Input: part model. Units: mm. Frame: model coordinates. A direction names the side the tool comes from. Give positions to 0.01 mm unless a question says otherwise; leave off trailing zeros. Loops run counter-clockwise (first coordinate to the right, second up) from the corner with the lowest first, then second, coordinate; pieces in that order, holes last. Notation, with made-up numbers: (23, 24.25) -> (32, 24.25) arc R27 cw to (32, 44.25) -> close; hole circle Ø4 at (29.25, 4.5). An arc over 180 degrees is marked (long way). Answer as a JSON object with one key per item and string values.
```python
from build123d import *

# Parameters (mm, degrees)
EXTRUDE1_DEPTH     = 53
HOLE1_D            = 9
HOLE1_DEPTH        = 53
SKETCH5_R          = 4
CUT_EXTRUDE1_DEPTH = 4
SKETCH6_R          = 5.5
CUT_EXTRUDE2_DEPTH = 3
SKETCH7_R          = 2
CUT_EXTRUDE3_DEPTH = 33
CUT_EXTRUDE4_DEPTH = 5


with BuildPart() as part:
    # Sketch1 → Extrude1 (new body)
    with BuildSketch(Plane(origin=(0, 0, 0), x_dir=(1, 0, 0), z_dir=(0, 1, 0))):
        with BuildLine():
            Line((-37.947331922, 31), (37.947331922, 31))
            ThreePointArc((37.947331922, 31), (49, 0), (37.947331922, -31))
            Line((37.947331922, -31), (-37.947331922, -31))
            ThreePointArc((-37.947331922, -31), (-49, 0), (-37.947331922, 31))
        make_face()
    extrude(amount=EXTRUDE1_DEPTH)

    # Sketch2 → Revolve1 (revolve)
    with BuildSketch(Plane.XY, mode=Mode.PRIVATE) as revolve1_sk:
        Polygon((0, 89), (-6.75, 89), (-6.75, 75), (-18, 75), (-18, 74), (-30.95, 74), (-30.95, 53), (0, 53), align=None)
    revolve(revolve1_sk.sketch.rotate(Axis((0, 0, 0), (0, 1, 0)), 270), axis=Axis((0, 0, 0), (0, 1, 0)))  # turned: the seam where the file's is

    # Hole1
    with Locations(Plane(origin=(0, 53, 0), x_dir=(-1, 0, 0), z_dir=(0, 1, 0))):
        with Locations((40, 0), (-40, 0)):
            Hole(HOLE1_D / 2, depth=HOLE1_DEPTH)

    # Sketch5 → Cut-Extrude1 (cut)
    with BuildSketch(Plane.XZ):
        with Locations(Location((0, 0, 0), (0, 0, 270))):  # turned: the seam where the file's is
            Circle(SKETCH5_R)
    extrude(amount=-CUT_EXTRUDE1_DEPTH, mode=Mode.SUBTRACT)

    # Sketch6 → Cut-Extrude2 (cut)
    with BuildSketch(Plane.XZ):
        with Locations(Location((31, -13, 0), (0, 0, 270))):  # turned: the seam where the file's is
            Circle(SKETCH6_R)
    extrude(amount=-CUT_EXTRUDE2_DEPTH, mode=Mode.SUBTRACT)

    # Sketch7 → Cut-Extrude3 (cut)
    with BuildSketch(Plane.XZ.offset(-3)):
        with Locations(Location((31, -13, 0), (0, 0, 270))):  # turned: the seam where the file's is
            Circle(SKETCH7_R)
    extrude(amount=-CUT_EXTRUDE3_DEPTH, mode=Mode.SUBTRACT)

    # Sketch8 → Cut-Revolve1 (revolve, cut)
    with BuildSketch(Plane(origin=(0, 0, 0), x_dir=(0.920504853, 0, -0.390731128), z_dir=(0.390731128, 0, 0.920504853)), mode=Mode.PRIVATE) as cut_revolve1_sk:
        Polygon((49, 28), (47, 28), (47, 33.4215), (45.517364509, 34.2775), (32, 34.2775), (32, 40), (49, 40), align=None)
    revolve(cut_revolve1_sk.sketch.rotate(Axis((47.484793311, 40, -20.156098913), (-0.920504853, 0, 0.390731128)), 270), axis=Axis((47.484793311, 40, -20.156098913), (-0.920504853, 0, 0.390731128)), mode=Mode.SUBTRACT)  # turned: the seam where the file's is

    # Sketch9 → Revolve2 (revolve)
    with BuildSketch(Plane(origin=(0, 0, 0), x_dir=(0.920504853, 0, -0.390731128), z_dir=(0.390731128, 0, 0.920504853)), mode=Mode.PRIVATE) as revolve2_sk:
        Polygon((47, 31), (47, 34.2775), (38, 34.2775), (37, 35.2775), (37, 40), (52, 40), (52, 31), align=None)
    revolve(revolve2_sk.sketch.rotate(Axis((53.930450878, 40, -22.892118224), (-0.920504853, 0, 0.390731128)), 270), axis=Axis((53.930450878, 40, -22.892118224), (-0.920504853, 0, 0.390731128)))  # turned: the seam where the file's is

    # Sketch10 → Cut-Extrude4 (cut)
    with BuildSketch(Plane(origin=(47.86625238, 0, -20.318018681), x_dir=(-0.390731128, 0, -0.920504853), z_dir=(0.920504853, 0, -0.390731128))):
        Polygon((4.041451884, 40), (2.020725942, 43.5), (-2.020725942, 43.5), (-4.041451884, 40), (-2.020725942, 36.5), (2.020725942, 36.5), align=None)
    extrude(amount=-CUT_EXTRUDE4_DEPTH, mode=Mode.SUBTRACT)


solid = part.part
```
Q1. Section C-C, the plane x = -40. Return the cut outline in (y, z), then the cut area to 3 significant figures.
Evaluation:
{"outline": "(0, -28.3) -> (53, -28.3) -> (53, -4.5) -> (0, -4.5) -> close; (0, 4.5) -> (53, 4.5) -> (53, 28.3) -> (0, 28.3) -> close", "area": "2,520 mm2"}
Q2. Pin query (flat end, axial travel): pin 1 (10 mm diameter, centred on x = 31, z = -13, fed in from +Y); pin 2 (5.5 mm diameter, centred on x = 32, z = -12.5, fed in from -Y); pin 3 (5.5 mm diameter, centred on x = -40, z = 0, fed in from +Y); pin 4 (4.5 mm diameter, centred on x = 31, z = -13, fed in from +Y). Return the tip coordinate at first contact, or that it passes through.
Evaluation:
{"pin 1": "stops at y = 74", "pin 2": "stops at y = 3", "pin 3": "passes through", "pin 4": "stops at y = 53"}
Q3. Access query for faces 4 (the flat face through (44.407, 41.726, -22.158)), 5 (the flat face through (28.6, 3, -12.9)), 6 (the flat face through (43.286, 40.049, -18.312)), 7 (the cylindrical face through (6.59, 81.9, 1.46)), 8 (the cylindrical face through (-35.708, 26.129, 1.352)). Directions: +Z, -Z, +X, -X, +Y, -Y. A direction counts if a zero-diameter tool reaches every point of the face in a straight line with its end or side. Return the directions, or none.
Evaluation:
{"face 4": "+X", "face 5": "-Y", "face 6": "none", "face 7": "+Y", "face 8": "+Y, -Y"}
Q4. Section D-D, the plane z = 21. Return the cut outline in (x, y), then the cut area to 3 significant figures.
Evaluation:
{"outline": "(-44.27, 0) -> (44.27, 0) -> (44.27, 53) -> (22.74, 53) -> (22.74, 74) -> (-22.74, 74) -> (-22.74, 53) -> (-44.27, 53) -> close", "area": "5,650 mm2"}
Q5. Section B-B, the plane x = 0. Return the cut outline in (y, z).
Evaluation:
{"outline": "(0, -31) -> (53, -31) -> (53, -30.95) -> (74, -30.95) -> (74, -18) -> (75, -18) -> (75, -6.75) -> (89, -6.75) -> (89, 6.75) -> (75, 6.75) -> (75, 18) -> (74, 18) -> (74, 30.95) -> (53, 30.95) -> (53, 31) -> (0, 31) -> (0, 4) -> (4, 4) -> (4, -4) -> (0, -4) -> close"}
Q6. Section A-A, the plane z = 0. Return the cut outline in (x, y).
Evaluation:
{"outline": "(-49, 0) -> (-44.5, 0) -> (-44.5, 53) -> (-49, 53) -> close; (-35.5, 0) -> (-4, 0) -> (-4, 4) -> (4, 4) -> (4, 0) -> (35.5, 0) -> (35.5, 53) -> (30.95, 53) -> (30.95, 74) -> (18, 74) -> (18, 75) -> (6.75, 75) -> (6.75, 89) -> (-6.75, 89) -> (-6.75, 75) -> (-18, 75) -> (-18, 74) -> (-30.95, 74) -> (-30.95, 53) -> (-35.5, 53) -> close; (44.5, 0) -> (49, 0) -> (49, 53) -> (44.5, 53) -> close"}
Q7. Ray query, line 1 along X through (y, z) = (32, -0.5); line 2 along Z through (x, y) = (31, 28); line 3 along Y through (x, z) = (-32, -2.5). Return the intervals inside material, ascending.
Evaluation:
{"line 1": "x = -49 to -44.47, -35.53 to 35.53, 44.47 to 49", "line 2": "z = -31 to -15, -11 to 31", "line 3": "y = 0 to 53"}
Q8. Draft query along Y for faces 1 (the flat face through (0, 89, 0)), 2 (the cylindrical face through (45.991, 31.077, -18.249)), 3 (the flat face through (1, 26, 31)). Return one class per face: +Y half, -Y half, draft (parallel to the pull), parting line (faces both ways), or undercut.
Evaluation:
{"face 1": "+Y half", "face 2": "undercut", "face 3": "draft"}
